```python
from build123d import *

# Parameters (mm, degrees)
BOSS_EXTRUDE2_DEPTH = 130
SKETCH3_W           = 6.156004655
SKETCH3_H           = 2
BOSS_EXTRUDE3_DEPTH = 10
SKETCH4_W           = 6.077661346
SKETCH4_H           = 2
BOSS_EXTRUDE4_DEPTH = 6
SKETCH5_R           = 1.5875
CUT_EXTRUDE1_DEPTH  = 132.968640925


with BuildPart() as part:
    # Sketch2 → Boss-Extrude2 (new body)
    with BuildSketch(Plane(origin=(0, 0, 0), x_dir=(0, 0, -1), z_dir=(1, 0, 0))):
        with BuildLine():
            Line((-0.835960879, 1.603184904), (-20.29416291, 3.210740854))
            ThreePointArc((-20.29416291, 3.210740854), (-22.509098324, 1.210740854), (-20.29416291, -0.789259146))
            Line((-20.29416291, -0.789259146), (-0.835960879, 1.603184904))
        make_face()
    extrude(amount=BOSS_EXTRUDE2_DEPTH)

    # Sketch3 → Boss-Extrude3 (add)
    with BuildSketch(Plane.ZY):
        with Locations((17.625252135, 1.210740854)):
            Rectangle(SKETCH3_W, SKETCH3_H)
    extrude(amount=BOSS_EXTRUDE3_DEPTH)

    # Sketch4 → Boss-Extrude4 (add)
    with BuildSketch(Plane(origin=(0, 0, 14.547249808), x_dir=(-1, 0, 0), z_dir=(0, 0, -1))):
        with Locations((6.961169327, 1.210740854)):
            Rectangle(SKETCH4_W, SKETCH4_H)
    extrude(amount=BOSS_EXTRUDE4_DEPTH)

    # Sketch5 → Cut-Extrude1 (cut, through all)
    with BuildSketch(Plane(origin=(0, 2.210740854, 0), x_dir=(1, 0, 0), z_dir=(0, 1, 0))):
        with Locations(Location((-7.057411019, -18.017090399, 0), (0, 0, 270))):
            Circle(SKETCH5_R)
    extrude(amount=-CUT_EXTRUDE1_DEPTH, mode=Mode.SUBTRACT)


solid = part.part
```
Build history of the part. All positions in model axes, mm. A direction names the side the tool comes from. Coordinates: 2 decimals unless noted, no trailing zeros. Order: outer loops, then holes, each group sorted by start corner. A loop starts at its lowest first (then second) coordinate and runs counter-clockwise, first axis right, second up. Notation, with made-up numbers: (60.25, -21) -> (110.25, -21) arc R23 ccw to (110.25, -8) -> close; hole circle Ø11 at (38.5, -24.5). An arc over 180 degrees is marked (long way). Answer in a Markdown table with one row per item. Add a question column.
Q1. Which spindle directions (+Z, -Z, +X, -X, +Y, -Y) get a long thin tool onto all of the face, cutting with end or side? Do faces 4 (the face through (64.09, 2.396, 10.429)), 5 (the face through (-5, 0.211, 15)), 6 (the face through (-5, 2.211, 15)). Say none if no direction does.
Q2. Mould opens along X. For faces 1 (the face through (64.09, 1.26, 22.51)), 2 (the face through (0, 1, 14)), 3 (the face through (130, 1, 14)) say: +X half, -X half, draft (parallel to the pull), parting line (faces both ways), or undercut.
Q3. Wall check: line 1 along X through (y, z) = (1.75, 12); line 2 along X through (y, z) = (0.15, 18.25); line 3 along X through (y, z) = (0.35, 9.5). Give the ranges that are in metal, low to high. Write a range as [from, to].
Q4. Band-saw the part on A-A, the plane x = 66.5. List the corners of the cut face in (y, z), then the cut area to 3 significant figures.
Q5. Drop flat-ended pins along their axis: pin 1 (8 mm diameter, centred on x = -7.5, z = 16, fed in from -Y); pin 2 (8 mm diameter, centred on x = 56, z = 11.5, fed in from +Y); pin 3 (2 mm diameter, centred on x = 42.5, y = 2, fed in from -Z); pin 4 (1.2 mm diameter, centred on y = 0.5, z = 8, fed in from -X). Give the stop position or say it passes through.
Answers follow:
| question | item | result |
|---|---|---|
| 1 | face 4 | -Z, +X, -X, +Y |
| 1 | face 5 | +Z, -Z, -X, -Y |
| 1 | face 6 | +Z, -Z, -X, +Y |
| 2 | face 1 | draft |
| 2 | face 2 | undercut |
| 2 | face 3 | +X half |
| 3 | line 1 | [-10, -3.92], [0, 130] |
| 3 | line 2 | [0, 130] |
| 3 | line 3 | [-10, -3.92] |
| 4 | outline | (-0.79, 20.29) -> (1.6, 0.84) -> (3.21, 20.29) arc R2.01 ccw (long way) to start |
| 4 | area | 46.1 mm^2 |
| 5 | pin 1 | y = 0.21 |
| 5 | pin 2 | y = 2.81 |
| 5 | pin 3 | z = 0.84 |
| 5 | pin 4 | x = -10 |
